Verification items for this drawing (mm, ordinates from the low corner). A direction names the side the tool comes from. Coordinates: 2 decimals unless noted, no trailing zeros. Order: outer loops, then holes, each group sorted by start corner. A loop starts at its lowest first (then second) coordinate and runs counter-clockwise, first axis right, second up. Notation, with made-up numbers: (77, 49) -> (123, 49) arc R16 cw to (123, 57) -> close; hole circle Ø11 at (9.25, 56.25). An arc over 180 degrees is marked (long way). Write item = value, one per line. Start each with the question number.
1. Cross-section at C-C on y = 38.5. Record the cut outline in (x, z).
2. Cross-section at B-B on z = 58. Record the cut outline in (x, y), plus the area to 3 significant figures.
3. Cross-section at A-A on y = 62. Record the cut outline in (x, z), plus the area to 3 significant figures.
4. Set-up check for the marked faces 1, 2, 3 and 4: record each of +Z, -Z, +X, -X, +Y, -Y from which the full face is reachable in a straight line by a thin tool's end or side.
5. Go/stop test with flat-tipped pins: P1, Ø9.5, axis at x = 13, y = 61.5, coming from the -Z side; P2, Ø2, axis at x = 46, y = 61, coming from the +Z side; P3, Ø6.5, axis at x = 34, y = 29.5, coming from the -Z side; P4, Ø9.5, axis at x = 50, y = 60, coming from the +Z side. Record where each tip stops, or that it passes through.
6. Thickness scan on line 1 along Y through (x, z) = (32, 50); line 2 along Z through (x, y) = (12, 64); line 3 along Z through (x, y) = (24, 16). Record the ranges inside material, lowest first. Write a range as from..to.
7. Cross-section at D-D on x = 13.5. Record the cut outline in (y, z), plus the area to 3 significant figures.
8. Release check for a two-part mould opening along Z. For the marked faces 5, 6 and 7 record: +Z half, -Z half, draft (parallel to the pull), parting line (faces both ways), or undercut.
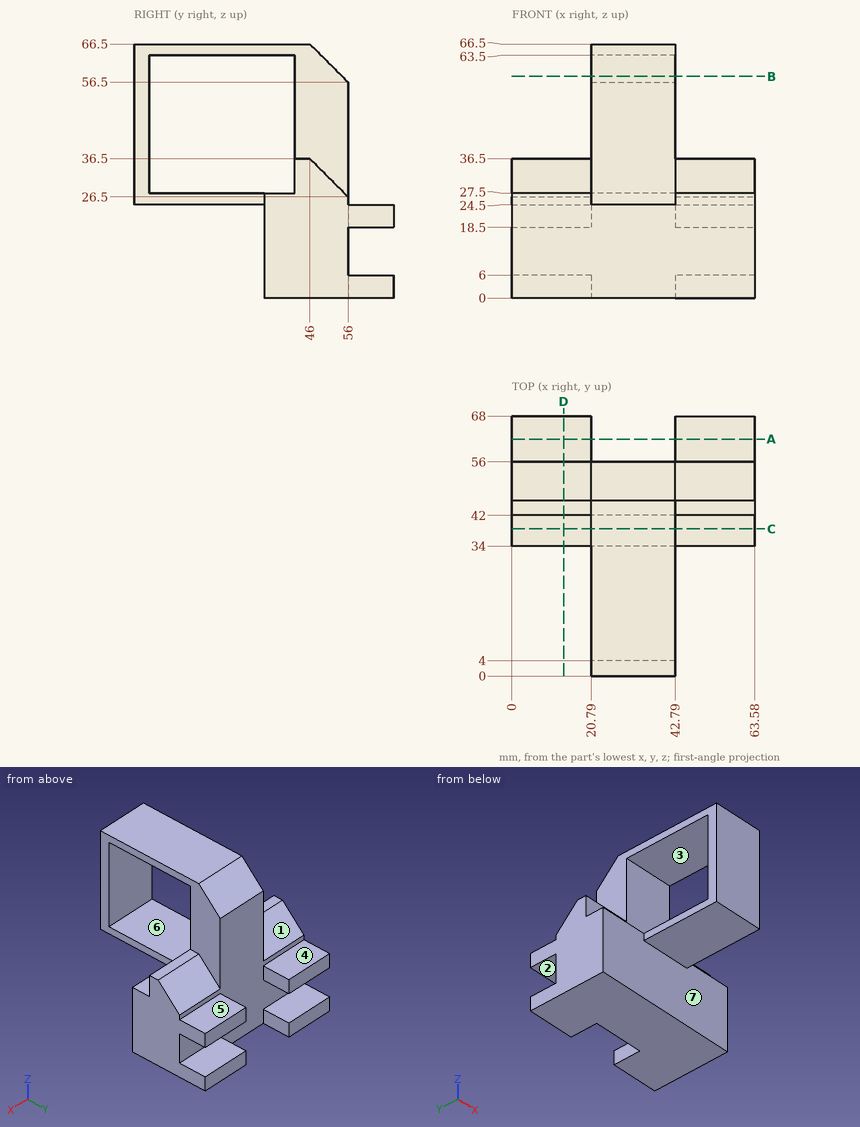
Worked out:
q1.outline = (0, 0) -> (63.58, 0) -> (63.58, 27.5) -> (0, 27.5) -> close; (20.79, 63.5) -> (42.79, 63.5) -> (42.79, 66.5) -> (20.79, 66.5) -> close
q2.outline = (20.79, 0) -> (42.79, 0) -> (42.79, 4) -> (20.79, 4) -> close; (20.79, 42) -> (42.79, 42) -> (42.79, 54.5) -> (20.79, 54.5) -> close
q2.area = 363 mm²
q3.outline = (0, 0) -> (20.79, 0) -> (20.79, 6) -> (0, 6) -> close; (0, 18.5) -> (20.79, 18.5) -> (20.79, 24.5) -> (0, 24.5) -> close; (42.79, 0) -> (63.58, 0) -> (63.58, 6) -> (42.79, 6) -> close; (42.79, 18.5) -> (63.58, 18.5) -> (63.58, 24.5) -> (42.79, 24.5) -> close
q3.area = 499 mm²
q4.face_1 = +Z, -X, +Y
q4.face_2 = +X, -X, +Y
q4.face_3 = +X, -X
q4.face_4 = +Z, +X, -X, +Y
q5.P1 = 0
q5.P2 = 24.5
q5.P3 = 24.5
q5.P4 = 27.25
q6.line_1 = 0..4, 42..56
q6.line_2 = 0..6, 18.5..24.5
q6.line_3 = 24.5..27.5, 63.5..66.5
q7.outline = (34, 0) -> (68, 0) -> (68, 6) -> (56, 6) -> (56, 18.5) -> (68, 18.5) -> (68, 24.5) -> (56, 24.5) -> (56, 26.5) -> (46, 36.5) -> (42, 36.5) -> (42, 27.5) -> (34, 27.5) -> close
q7.area = 825 mm²
q8.face_5 = +Z half
q8.face_6 = undercut
q8.face_7 = draft
